from build123d import *

# Parameters (mm, degrees)
SKETCH1_R           = 8.8
SKETCH1_R_2         = 3
BOSS_EXTRUDE1_DEPTH = 18.5
SKETCH2_OUTSIDE_W   = 25.802
SKETCH2_OUTSIDE_H   = 25.802
SKETCH2_OUTSIDE_R   = 4.5
CUT_EXTRUDE1_DEPTH  = 6.5
SKETCH3_OUTSIDE_W   = 25.802
SKETCH3_OUTSIDE_H   = 25.802
SKETCH3_OUTSIDE_R   = 4.5
CUT_EXTRUDE2_DEPTH  = 6.5
SKETCH4_OUTSIDE_W   = 25.802
SKETCH4_OUTSIDE_H   = 25.802
SKETCH4_OUTSIDE_R   = 6.8
CUT_EXTRUDE3_DEPTH  = 3.5
CUT_EXTRUDE4_START  = -1
SKETCH5_OUTSIDE_W   = 25.802
SKETCH5_OUTSIDE_H   = 25.802
SKETCH5_OUTSIDE_R   = 6
CUT_EXTRUDE4_DEPTH  = 1
CHAMFER1_SIZE       = 0.5


with BuildPart() as part:
    # Sketch1 → Boss-Extrude1 (new body)
    with BuildSketch(Plane.XY):
        Circle(SKETCH1_R)
        Circle(SKETCH1_R_2, mode=Mode.SUBTRACT)
    extrude(amount=BOSS_EXTRUDE1_DEPTH)

    # Sketch2 outside → Cut-Extrude1 (cut)
    with BuildSketch(Plane.XY.offset(18.5)):
        Rectangle(SKETCH2_OUTSIDE_W, SKETCH2_OUTSIDE_H)
        Circle(SKETCH2_OUTSIDE_R, mode=Mode.SUBTRACT)
    extrude(amount=-CUT_EXTRUDE1_DEPTH, mode=Mode.SUBTRACT)

    # Sketch3 outside → Cut-Extrude2 (cut)
    with BuildSketch(Plane(origin=(0, 0, 0), x_dir=(-1, 0, 0), z_dir=(0, 0, -1))):
        Rectangle(SKETCH3_OUTSIDE_W, SKETCH3_OUTSIDE_H)
        with Locations(Location((0, 0, 0), (0, 0, 180))):
            Circle(SKETCH3_OUTSIDE_R, mode=Mode.SUBTRACT)
    extrude(amount=-CUT_EXTRUDE2_DEPTH, mode=Mode.SUBTRACT)

    # Sketch4 outside → Cut-Extrude3 (cut)
    with BuildSketch(Plane.XY.offset(12)):
        Rectangle(SKETCH4_OUTSIDE_W, SKETCH4_OUTSIDE_H)
        Circle(SKETCH4_OUTSIDE_R, mode=Mode.SUBTRACT)
    extrude(amount=-CUT_EXTRUDE3_DEPTH, mode=Mode.SUBTRACT)

    # Sketch5 outside → Cut-Extrude4 (cut)
    with BuildSketch(Plane.XY.offset(12).offset(CUT_EXTRUDE4_START)):
        Rectangle(SKETCH5_OUTSIDE_W, SKETCH5_OUTSIDE_H)
        Circle(SKETCH5_OUTSIDE_R, mode=Mode.SUBTRACT)
    extrude(amount=-CUT_EXTRUDE4_DEPTH, mode=Mode.SUBTRACT)

    # Chamfer1
    chamfer1_edges = [part.edges().sort_by_distance(p)[0] for p in [
        (-4.5, 0, 18.5),
        (-4.5, 0, 0),
    ]]
    chamfer(chamfer1_edges, length=CHAMFER1_SIZE)


solid = part.part
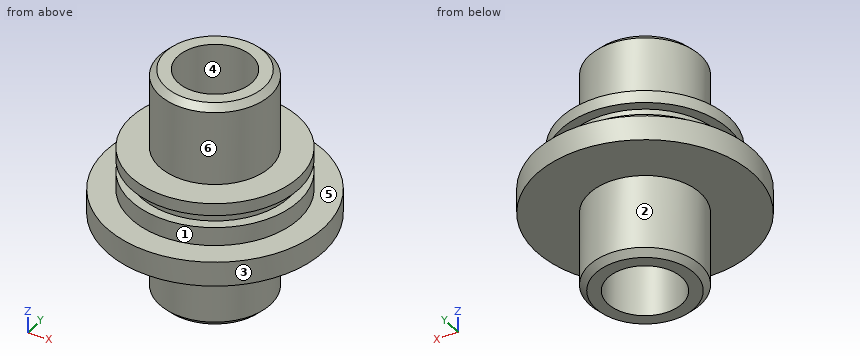
For this review, take the finished solid that the model builds, in its own axes (mm). Face numbers are marked on the shaded views. A direction names the side the tool comes from. Coordinates: 2 decimals unless noted, no trailing zeros. Loops run counter-clockwise (first coordinate to the right, second up) from the corner with the lowest first, then second, coordinate; pieces in that order, holes last. Notation, with made-up numbers: (-26.5, 61.25) - (-13.5, 61.25) arc R25 ccw to (-13.5, 81.25) - close; hole circle Ø1 at (7, -37). An arc over 180 degrees is marked (long way). Use a Markdown table: item, result. Add a question column.
Item 1: For line 1 (Y direction, x = 0, z = 7); line 2 (Y direction, x = 0, z = 5.25); line 3 (Z direction, x = -4.25, y = 4.5), list the stretches that pass through material, from the lowest coordinate up.
Item 2: Insertion check: pin 1 Ø3 at (y, z) = (-5.5, 15) entering from +X; pin 2 Ø2 at (x, z) = (-2.5, 6.5) entering from +Y; pin 3 Ø5 at (y, z) = (-3, 5.5) entering from +X. Each pin has a flat end and moves straight along its axis. Give the tip position at first contact, or say it passes through.
Item 3: We need section C-C (z = 2.25). Give the boundary of the cut face in (x, y), and give its area (3 significant figures).
Item 4: Tool access review of the marked faces 1, 2 and 3: name each direction out of +Z, -Z, +X, -X, +Y, -Y from which nothing blocks a thin tool from reaching the whole face with its end or side.
Item 5: Mouldability with a two-part tool opening along Y and no side actions: class the marked faces 4, 5 and 6 as pulls with the +Y half, pulls with the -Y half, needs draft (parallel to the pull), parting line crosses it, or undercut.
Item 6: We need section D-D (x = 5.5). Give the boundary of the cut face in (y, z), and give its area (3 significant figures).
Results list:
| question | item | result |
|---|---|---|
| 1 | line 1 | y = -8.8 to -3, 3 to 8.8 |
| 1 | line 2 | y = -4.5 to -3, 3 to 4.5 |
| 1 | line 3 | z = 6.5 to 10, 11 to 12 |
| 2 | pin 1 | stops at x = 2.06 |
| 2 | pin 2 | stops at y = 8.67 |
| 2 | pin 3 | stops at x = 8.77 |
| 3 | outline | circle Ø9 at (0, 0); hole circle Ø6 at (0, 0) |
| 3 | area | 35.3 mm^2 |
| 4 | face 1 | +Z |
| 4 | face 2 | -Z |
| 4 | face 3 | +Z, -Z |
| 5 | face 4 | undercut |
| 5 | face 5 | needs draft |
| 5 | face 6 | parting line crosses it |
| 6 | outline | (-6.87, 6.5) - (6.87, 6.5) - (6.87, 8.5) - (4, 8.5) - (4, 10) - (2.4, 10) - (2.4, 11) - (4, 11) - (4, 12) - (-4, 12) - (-4, 11) - (-2.4, 11) - (-2.4, 10) - (-4, 10) - (-4, 8.5) - (-6.87, 8.5) - close |
| 6 | area | 52.3 mm^2 |
